from build123d import *

# Parameters (mm, degrees)
F2_SIZE  = 1
F3_R     = 2.99999
F5_DEPTH = 30


# Not quite as in the source:
# - a fillet or chamfer is up to 0.001 mm smaller than in the source, because OpenCascade refuses the exact size


with BuildPart() as f1:
    # F0 (on Front) → F1 (revolve)
    with BuildSketch(Plane.XZ):
        Polygon((10, 30), (10, 0), (20, 0), (20, 14), (28.5, 14), (33, 14.7934714132), (33, 26), (20.5, 26), (20.5, 30), align=None)
    revolve(axis=Axis((0, 0, 2.9418331105), (0, 0, 1)))

    # F2
    f2_edges = [f1.edges().sort_by_distance(p)[0] for p in [
        (-20.5, 0, 30),
        (-33, 0, 26),
        (-20, 0, 0),
        (-10, 0, 30),
        (-10, 0, 0),
    ]]
    chamfer(f2_edges, length=F2_SIZE)

    # F3 (radius 3 in the source; OpenCascade refuses exactly that, so slightly less here)
    f3_edges = [f1.edges().sort_by_distance(p)[0] for p in [
        (-20, 0, 14),
        (-20.5, 0, 26),
    ]]
    fillet(f3_edges, radius=F3_R)

    # F4 (on face) → F5 (cut, through all)
    with BuildSketch(Plane.XY.offset(30)):
        with BuildLine():
            Line((2.5, 13.5), (-2.5, 13.5))
            Line((-2.5, 13.5), (-2.5, 10.7121426428))
            ThreePointArc((-2.5, 10.7121426428), (0, 11), (2.5, 10.7121426428))
            Line((2.5, 10.7121426428), (2.5, 13.5))
        make_face()
        with BuildLine():
            ThreePointArc((2.5, 10.7121426428), (0, 11), (-2.5, 10.7121426428))
            Line((-2.5, 10.7121426428), (-2.5, 9.6824583655))
            ThreePointArc((-2.5, 9.6824583655), (0, 10), (2.5, 9.6824583655))
            Line((2.5, 9.6824583655), (2.5, 10.7121426428))
        make_face()
    extrude(amount=-F5_DEPTH, mode=Mode.SUBTRACT)


solid = f1.part
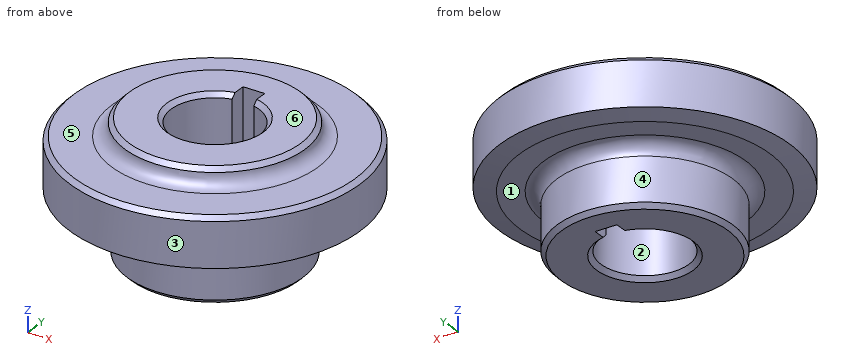
Could you check a few things on this model? Use its own coordinates, in mm. Face numbers are marked on the shaded views. A direction names the side the tool comes from. Give positions to 0.01 mm unless a question says otherwise; leave off trailing zeros. Write each loop counter-clockwise with the first axis right and the second up, starting at its lowest first coordinate (ties: lowest second). Pieces come first, ordered by that corner, then holes. Notation, with made-up numbers: (38.5, 69) -> (70.5, 69) arc R13 ccw to (70.5, 82) -> close; hole circle Ø8 at (1.5, 21). An arc over 180 degrees is marked (long way). Answer as a JSON object with one key per item and string values.
Q1. Please list where these lines run through material, in increasing order: L1, parallel to Y at x = 0, z = 7; L2, parallel to Y at x = 0.5, z = 23; L3, parallel to X at y = 3.5, z = 20.5.
Taken from the geometry:
{"L1": "y = -20 to -10, 13.5 to 20", "L2": "y = -33 to -9.99, 13.5 to 33", "L3": "x = -32.81 to -9.37, 9.37 to 32.81"}
Q2. We'd pull the mould along Y, two halves only. Please class the marked faces 1, 2 and 3: released by +Y, released by -Y, zero draft, split by the parting line, or undercut.
Taken from the geometry:
{"face 1": "zero draft", "face 2": "undercut", "face 3": "split by the parting line"}
Q3. Will these pins go through, and if not, where does the flat tip stop? pin 1 Ø5 at (x, y) = (25.5, -22) entering from -Z; pin 2 Ø8 at (x, z) = (-25, 17.5) entering from +Y; pin 3 Ø1.5 at (x, z) = (-0.5, 9.5) entering from -Y.
Taken from the geometry:
{"pin 1": "stops at z = 14.47", "pin 2": "stops at y = 25.46", "pin 3": "stops at y = -20"}
Q4. Suppose I cut it at B-B on z = 19.5. Write out the boundary of the cut face in (x, y), then the cut area to 3 significant figures.
Taken from the geometry:
{"outline": "circle Ø66 at (0, 0); hole (-2.5, 9.68) arc R10 ccw (long way) to (2.5, 9.68) -> (2.5, 13.5) -> (-2.5, 13.5) -> close", "area": "3,090 mm²"}
Q5. Which directions (+Z, -Z, +X, -X, +Y, -Y) give clear straight access to the entire face, cutting with the end or side of a thin tool? Please do the marked faces 4, 5 and 6.
Taken from the geometry:
{"face 4": "-Z", "face 5": "+Z", "face 6": "+Z, +X, -X, +Y, -Y"}
Q6. Suppose I cut it at D-D on z = 27. Write out the boundary of the cut face in (x, y), then the cut area to 3 significant figures.
Taken from the geometry:
{"outline": "circle Ø42.53 at (0, 0); hole (-2.5, 9.68) arc R10 ccw (long way) to (2.5, 9.68) -> (2.5, 13.5) -> (-2.5, 13.5) -> close", "area": "1,090 mm²"}
